```python
from build123d import *

# Parameters (mm, degrees)
F0_R     = 2.65
F1_DEPTH = 4
F2_R     = 1.15
F3_DEPTH = 10


with BuildPart() as f1:
    # F0 (on Front) → F1 (new body)
    with BuildSketch(Plane.XZ):
        with BuildLine():
            Line((-7.5, -5), (7.5, -5))
            Line((7.5, -5), (7.5, 5))
            Line((7.5, 5), (-7.5, 5))
            ThreePointArc((-7.5, 5), (-12.5, 0), (-7.5, -5))
        make_face()
        with Locations((-7.5, 0)):
            Circle(F0_R, mode=Mode.SUBTRACT)
    extrude(amount=F1_DEPTH)

    # F2 (on face) → F3 (join, through all)
    with BuildSketch(Plane(origin=(0, 0, -5), x_dir=(1, 0, 0), z_dir=(0, 0, -1))):
        with BuildLine():
            Line((0, 4), (7.5, 4))
            Line((7.5, 4), (7.5, 10.48325))
            ThreePointArc((7.5, 10.48325), (3.75, 14.23325), (0, 10.48325))
            Line((0, 10.48325), (0, 4))
        make_face()
        with Locations((3.75, 10.48325)):
            Circle(F2_R, mode=Mode.SUBTRACT)
    extrude(amount=-F3_DEPTH)


solid = f1.part
```
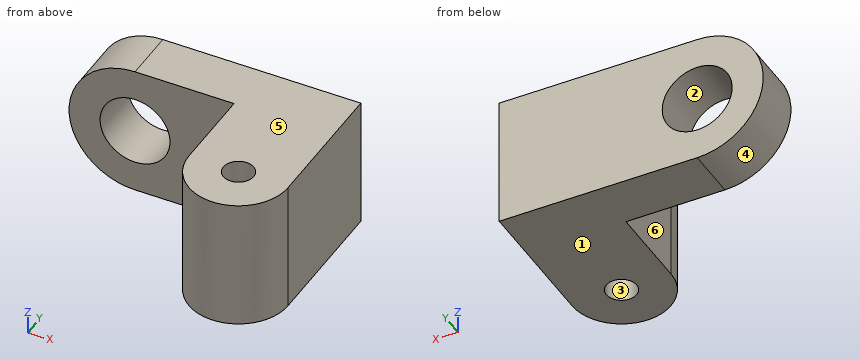
Input: part model. Units: mm. Frame: model coordinates. Face numbers are marked on the shaded views. A direction names the side the tool comes from. Coordinates: 2 decimals unless noted, no trailing zeros. Write each loop counter-clockwise with the first axis right and the second up, starting at its lowest first coordinate (ties: lowest second). Pieces come first, ordered by that corner, then holes.
1) Section D-D on z = -4. Output: boundary loops of the cut face in (x, y), and give its area (3 significant figures).
2) Material intervals for line 1 along Y through (x, z) = (3.75, 0.75); line 2 along Z through (x, y) = (-7.5, -1.85); line 3 along X through (y, z) = (-11.5, -2), sorted ascending.
3) Section C-C on y = -1.75. Output: boundary loops of the cut face in (x, z).
4) Set-up query: the marked faces 5 and 6. Return all of +Z, -Z, +X, -X, +Y, -Y with unobstructed straight access to the full face (end or side cutting, diameter ignored); none if empty.
5) Mould query, pull axis Z, two halves, no side actions, for the marked faces 1, 2, 3 and 4. Classes: pulls with the +Z half, pulls with the -Z half, needs draft (parallel to the pull), parting line crosses it, or undercut.
6) Section A-A on z = 0. Output: boundary loops of the cut face in (x, y), and give its area (3 significant figures).
7) Section B-B on x = -5.25. Output: boundary loops of the cut face in (y, z).
8) Pin query (flat end, axial travel): pin 1 Ø3 at (y, z) = (-8, 2) entering from -X; pin 2 Ø1.5 at (x, z) = (3, 1.5) entering from -Y; pin 3 Ø3 at (x, z) = (-5, -3.5) entering from -Y; pin 4 Ø1.5 at (x, y) = (-2.5, -10.5) entering from -Z. Return the tip coordinate at first contact, or that it passes through.
Check result:
1. outline: (-10.5, -4) - (0, -4) - (0, -10.48) arc R3.75 ccw to (7.5, -10.48) - (7.5, 0) - (-10.5, 0) - close; hole circle Ø2.3 at (3.75, -10.48)
1. area: 139 mm2
2. line 1: y = -14.23 to -11.63, -9.33 to 0
2. line 2: z = -5 to -2.65, 2.65 to 5
2. line 3: x = 0.14 to 3.21, 4.29 to 7.36
3. outline: (-7.5, -5) - (7.5, -5) - (7.5, 5) - (-7.5, 5) arc R5 ccw to start; hole circle Ø5.3 at (-7.5, 0)
4. face 5: +Z, +X, -X, +Y, -Y
4. face 6: +Z, -Z, -X, -Y
5. face 1: pulls with the -Z half
5. face 2: undercut
5. face 3: needs draft
5. face 4: parting line crosses it
6. outline: (-12.5, -4) - (-10.15, -4) - (-10.15, 0) - (-12.5, 0) - close; (-4.85, -4) - (0, -4) - (0, -10.48) arc R3.75 ccw to (7.5, -10.48) - (7.5, 0) - (-4.85, 0) - close; hole circle Ø2.3 at (3.75, -10.48)
6. area: 125 mm2
7. outline: (-4, -5) - (0, -5) - (0, -1.4) - (-4, -1.4) - close; (-4, 1.4) - (0, 1.4) - (0, 5) - (-4, 5) - close
8. pin 1: stops at x = 0
8. pin 2: stops at y = -14.23
8. pin 3: stops at y = -4
8. pin 4: passes through
